```python
from build123d import *

# Parameters (mm, degrees)
F0_W        = 20
F0_H        = 10
F0_W_2      = 17.7
F0_H_2      = 7.5
F0_R        = 2.5
F0_R_2      = 1.5
F1_DEPTH    = 20
F2_DEPTH    = 5
F3_SIZE2    = 10
F3_SIZE     = 1
F4_T1_DEPTH = 22.5249378106
F4_T3_DEPTH = 12.5249378106
F4_T5_DEPTH = 25
F4_T7_DEPTH = 15


# Not quite as in the source:
# - a fillet or chamfer that OpenCascade refuses, or shapes differently, is made with other operations: its cross-section is extruded or revolved along the edge and cut away or added


with BuildPart() as f1:
    # F0 (on Top) → F1 (new body)
    with BuildSketch(Plane.XY):
        Rectangle(F0_W, F0_H)
        Rectangle(F0_W_2, F0_H_2, mode=Mode.SUBTRACT)
        Rectangle(F0_W_2, F0_H_2)
        with Locations((-5, 0)):
            Circle(F0_R, mode=Mode.SUBTRACT)
        with Locations((5, 0)):
            Circle(F0_R, mode=Mode.SUBTRACT)
        with Locations((5, 0)):
            Circle(F0_R)
        with Locations((5, 0)):
            Circle(F0_R_2, mode=Mode.SUBTRACT)
        with Locations((-5, 0)):
            Circle(F0_R)
        with Locations((-5, 0)):
            Circle(F0_R_2, mode=Mode.SUBTRACT)
    extrude(amount=F1_DEPTH)

    # F0 (on Top) → F2 (cut)
    with BuildSketch(Plane.XY):
        with Locations((-5, 0)):
            Circle(F0_R)
        with Locations((-5, 0)):
            Circle(F0_R_2, mode=Mode.SUBTRACT)
        with Locations((5, 0)):
            Circle(F0_R)
        with Locations((5, 0)):
            Circle(F0_R_2, mode=Mode.SUBTRACT)
    extrude(amount=F2_DEPTH, mode=Mode.SUBTRACT)

    # F3
    f3_edges = [f1.edges().sort_by_distance(p)[0] for p in [
        (0, -5, 0),
        (-10, 0, 0),
        (0, 5, 0),
        (10, 0, 0),
    ]]
    f3_side = f1.faces().sort_by_distance((0, 0, 0))[0]
    chamfer(f3_edges, length=F3_SIZE, length2=F3_SIZE2, reference=f3_side)

    # F4: fillet of radius 1 on 12 edges, made by hand

    # F4_s2 → F4_t1 (cut)
    with BuildSketch(Plane.YZ.offset(-11.2624689053)):
        with BuildLine():
            ThreePointArc((-3.0950124379, 0), (-3.7660177586, 0.2585474664), (-4.0900496281, 0.900496281))
            Line((-4.0900496281, 0.900496281), (-4, 0))
            Line((-4, 0), (-3.0950124379, 0))
        make_face()
        with BuildLine():
            ThreePointArc((4.0900496281, 0.900496281), (3.7660177586, 0.2585474664), (3.0950124379, 0))
            Line((3.0950124379, 0), (4, 0))
            Line((4, 0), (4.0900496281, 0.900496281))
        make_face()
    extrude(amount=F4_T1_DEPTH, mode=Mode.SUBTRACT)

    # F4_s4 → F4_t3 (cut)
    with BuildSketch(Plane.XZ.offset(-6.2624689053)):
        with BuildLine():
            ThreePointArc((-8.0950124379, 0), (-8.7660177586, 0.2585474664), (-9.0900496281, 0.900496281))
            Line((-9.0900496281, 0.900496281), (-9, 0))
            Line((-9, 0), (-8.0950124379, 0))
        make_face()
        with BuildLine():
            ThreePointArc((9.0900496281, 0.900496281), (8.7660177586, 0.2585474664), (8.0950124379, 0))
            Line((8.0950124379, 0), (9, 0))
            Line((9, 0), (9.0900496281, 0.900496281))
        make_face()
    extrude(amount=F4_T3_DEPTH, mode=Mode.SUBTRACT)

    # F4_s6 → F4_t5 (cut)
    with BuildSketch(Plane.YZ.offset(-12.5)):
        with BuildLine():
            ThreePointArc((-4, 20), (-4.7071067812, 19.7071067812), (-5, 19))
            Line((-5, 19), (-5, 20))
            Line((-5, 20), (-4, 20))
        make_face()
        with BuildLine():
            ThreePointArc((5, 19), (4.7071067812, 19.7071067812), (4, 20))
            Line((4, 20), (5, 20))
            Line((5, 20), (5, 19))
        make_face()
    extrude(amount=F4_T5_DEPTH, mode=Mode.SUBTRACT)

    # F4_s8 → F4_t7 (cut)
    with BuildSketch(Plane.XZ.offset(-7.5)):
        with BuildLine():
            ThreePointArc((10, 19), (9.7071067812, 19.7071067812), (9, 20))
            Line((9, 20), (10, 20))
            Line((10, 20), (10, 19))
        make_face()
        with BuildLine():
            ThreePointArc((-9, 20), (-9.7071067812, 19.7071067812), (-10, 19))
            Line((-10, 19), (-10, 20))
            Line((-10, 20), (-9, 20))
        make_face()
    extrude(amount=F4_T7_DEPTH, mode=Mode.SUBTRACT)

    # F4_s9 → F4_t10 (revolve, cut)
    with BuildSketch(Plane.XZ):
        with BuildLine():
            ThreePointArc((7.5, 20), (6.7928932188, 19.7071067812), (6.5, 19))
            Line((6.5, 19), (6.5, 20))
            Line((6.5, 20), (7.5, 20))
        make_face()
    revolve(axis=Axis((5, 0, 20), (0, 0, 1)), mode=Mode.SUBTRACT)

    # F4_s11 → F4_t12 (revolve, cut)
    with BuildSketch(Plane.XZ):
        with BuildLine():
            ThreePointArc((-2.5, 20), (-3.2071067812, 19.7071067812), (-3.5, 19))
            Line((-3.5, 19), (-3.5, 20))
            Line((-3.5, 20), (-2.5, 20))
        make_face()
    revolve(axis=Axis((-5, 0, 20), (0, 0, 1)), mode=Mode.SUBTRACT)

    # F4_s13 → F4_t14 (revolve, cut)
    with BuildSketch(Plane.XZ):
        with BuildLine():
            ThreePointArc((8.5, 0), (7.7928932188, 0.2928932188), (7.5, 1))
            Line((7.5, 1), (7.5, 0))
            Line((7.5, 0), (8.5, 0))
        make_face()
    revolve(axis=Axis((5, 0, 0), (0, 0, 1)), mode=Mode.SUBTRACT)

    # F4_s15 → F4_t16 (revolve, cut)
    with BuildSketch(Plane.XZ):
        with BuildLine():
            ThreePointArc((-1.5, 0), (-2.2071067812, 0.2928932188), (-2.5, 1))
            Line((-2.5, 1), (-2.5, 0))
            Line((-2.5, 0), (-1.5, 0))
        make_face()
    revolve(axis=Axis((-5, 0, 0), (0, 0, 1)), mode=Mode.SUBTRACT)


solid = f1.part
```
Geometry: final body of the model. Coordinates: model frame, mm. A direction names the side the tool comes from. Coordinates: 2 decimals unless noted, no trailing zeros. Order: outer loops, then holes, each group sorted by start corner. A loop starts at its lowest first (then second) coordinate and runs counter-clockwise, first axis right, second up. Notation, with made-up numbers: M 60,-21.5 L 67,-21.5 A25 ccw 67,16.5 Z; hole C 88.5,-30 d7. An arc over 180 degrees is marked long. Answer in a Markdown table with one row per item. Add a question column.
Q1. Contact query for flat-ended pins moving along their axis: P1, Ø4, axis at x = -5, y = 0, coming from the -Z side; P2, Ø4, axis at x = -5, y = 0, coming from the +Z side; P3, Ø4, axis at x = -6, y = 0, coming from the -Z side; P4, Ø5, axis at y = -3, z = 7.5, coming from the +X side. Output: stop coordinate, or through.
Q2. Section query B-B on y = 0. Count the separate pieces of the cut face and the enclosed holes in it, and give its area (3 significant figures).
Q3. Reachability of faces 5 (the flat face through (0, 0, 0)), 6 (the flat face through (-5, -2, 5)) from +Z, -Z, +X, -X, +Y, -Y: full face, straight path, thin tool, end or side. Return the list, or none.
Q4. Section query A-A on z = 13. Return the cut outline in (x, y), and give its area (3 significant figures).
Q5. Section query D-D on x = 5. Return the cut outline in (y, z).
Q6. Mould query, pull axis Y, two halves, no side actions, for faces 1 (the flat face through (-0.14, -4.55, 5.51)), 2 (the cylindrical face through (7.385, 0.751, 2.972)), 3 (the flat face through (-0.14, 4.55, 5.51)), 4 (the flat face through (10, 0, 14)). Classes: released by +Y, released by -Y, zero draft, split by the parting line, or undercut.
Q7. Section query C-C on x = 0.5. Return the cut outline in (y, z), and give its area (3 significant figures).
Q8. Line query: L1, parallel to Y at x = 5, z = 10.5; L2, parallel to X at y = -0.5, z = 1; L3, parallel to X at y = 0.5, z = 7.5. Output: solid intervals per line, ascending.
Completed:
| question | item | result |
|---|---|---|
| 1 | P1 | stops at z = 5 |
| 1 | P2 | stops at z = 19.87 |
| 1 | P3 | stops at z = 0.13 |
| 1 | P4 | stops at x = 10 |
| 2 | separate pieces | 3 |
| 2 | enclosed holes | 0 |
| 2 | area | 248 mm2 |
| 3 | face 5 | -Z, +X, -X, +Y, -Y |
| 3 | face 6 | -Z |
| 4 | outline | M -10,-5 L 10,-5 L 10,5 L -10,5 Z; hole C -5,0 d3; hole C 5,0 d3 |
| 4 | area | 186 mm2 |
| 5 | outline | M -5,10 L -4.09,0.9 A1 ccw -3.3,0.02 A1 ccw -2.5,1 L -2.5,5 L -1.5,5 L -1.5,19 A1 ccw -2.5,20 L -4,20 A1 ccw -5,19 Z; M 1.5,5 L 2.5,5 L 2.5,1 A1 ccw 3.3,0.02 A1 ccw 4.09,0.9 L 5,10 L 5,19 A1 ccw 4,20 L 2.5,20 A1 ccw 1.5,19 Z |
| 6 | face 1 | released by -Y |
| 6 | face 2 | undercut |
| 6 | face 3 | released by +Y |
| 6 | face 4 | zero draft |
| 7 | outline | M -5,10 L -4.09,0.9 A1 ccw -3.1,0 L 3.1,0 A1 ccw 4.09,0.9 L 5,10 L 5,19 A1 ccw 4,20 L -4,20 A1 ccw -5,19 Z |
| 7 | area | 189 mm2 |
| 8 | L1 | y = -5 to -1.5, 1.5 to 5 |
| 8 | L2 | x = -9.1 to -7.45, -2.55 to 2.55, 7.45 to 9.1 |
| 8 | L3 | x = -9.75 to -6.41, -3.59 to 3.59, 6.41 to 9.75 |
